```python
from build123d import *

# Parameters (mm, degrees)
F0_R     = 14.2875
F1_DEPTH = 14.2875
F2_R     = 6.35
F3_DEPTH = 44.45
F4_R     = 4.445
F5_DEPTH = 76.2


with BuildPart() as f1:
    # F0 (on Top) → F1 (new body, symmetric)
    with BuildSketch(Plane.XY):
        Circle(F0_R)
    extrude(amount=F1_DEPTH, both=True)

    # F2 (on face) → F3 (join)
    with BuildSketch(Plane(origin=(0, 0, -14.2875), x_dir=(1, 0, 0), z_dir=(0, 0, -1))):
        Circle(F2_R)
    extrude(amount=F3_DEPTH)

    # F4 (on Right) → F5 (join, symmetric)
    with BuildSketch(Plane.YZ):
        with Locations((0, -1.5875)):
            Circle(F4_R)
    extrude(amount=F5_DEPTH, both=True)

    # F6 (on Front) → F7 (revolve)
    with BuildSketch(Plane.XZ):
        with BuildLine():
            Line((-86.73837, -1.5875), (-66.41837, -1.5875))
            ThreePointArc((-66.41837, -1.5875), (-76.57837, 8.5725), (-86.73837, -1.5875))
        make_face()
        with BuildLine():
            ThreePointArc((86.73837, -1.5875), (76.57837, 8.5725), (66.41837, -1.5875))
            Line((66.41837, -1.5875), (86.73837, -1.5875))
        make_face()
    revolve(axis=Axis((-76.57837, 0, -1.5875), (-1, 0, 0)))


solid = f1.part
```
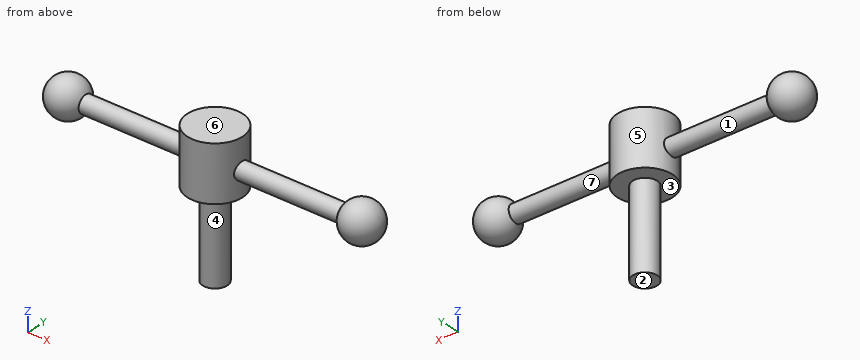
Here's how the part is built. I have some questions about the finished solid (model axes, mm). Face numbers are marked on the shaded views. A direction names the side the tool comes from. Coordinates: 2 decimals unless noted, no trailing zeros. Loops run counter-clockwise (first coordinate to the right, second up) from the corner with the lowest first, then second, coordinate; pieces in that order, holes last. Notation, with made-up numbers: M -24,-12 L 7,-12 A17 ccw 7,4 Z; hole C 59.25,-39 d4. An arc over 180 degrees is marked long. One line per item, written item: value.
1. On a 3-axis mill with a long thin cutter (end or side, diameter ignored), from which of +Z, -Z, +X, -X, +Y, -Y can I reach the whole of each face in a straight line? I mean the marked faces 1, 2 and 3. Say none if no direction works.
Geometry says:
face 1: none
face 2: -Z, +X, -X, +Y, -Y
face 3: -Z
2. Imagine slicing it at B-B (y = 0). List the corners of the cut face in (x, z) for me.
Geometry says:
outline: M -67.44,-6.03 L -14.29,-6.03 L -14.29,-14.29 L -6.35,-14.29 L -6.35,-58.74 L 6.35,-58.74 L 6.35,-14.29 L 14.29,-14.29 L 14.29,-6.03 L 67.44,-6.03 A10.16 ccw long 67.44,2.86 L 14.29,2.86 L 14.29,14.29 L -14.29,14.29 L -14.29,2.86 L -67.44,2.86 A10.16 ccw long Z
3. Imagine slicing it at A-A (x = 0). List the corners of the cut face in (y, z) for me.
Geometry says:
outline: M -14.29,-14.29 L -6.35,-14.29 L -6.35,-58.74 L 6.35,-58.74 L 6.35,-14.29 L 14.29,-14.29 L 14.29,14.29 L -14.29,14.29 Z
4. Imagine slicing it at C-C (z = -41). List the corners of the cut face in (x, y) for me.
Geometry says:
outline: C 0,0 d12.7
5. Thinking about a two-plate mould opening in X: for the marked faces 4, 5, 6 and 7, which applies, +X half, -X half, draft (parallel to the pull), parting line (faces both ways), or undercut?
Geometry says:
face 4: parting line
face 5: undercut
face 6: draft
face 7: undercut
6. Imagine slicing it at D-D (y = -8.25). List the corners of the cut face in (x, z) for me, and give its area (3 significant figures).
Geometry says:
outline: C -76.58,-1.59 d11.86; M -11.66,-14.29 L 11.66,-14.29 L 11.66,14.29 L -11.66,14.29 Z; C 76.58,-1.59 d11.86
area: 888 mm2
7. Will these pins go through, and if not, where does the flat tip stop? pin 1 Ø4 at (y, z) = (1, -1) entering from +X; pin 2 Ø4 at (y, z) = (-6.5, -18) entering from +X; pin 3 Ø1 at (y, z) = (-7, -2) entering from +X; pin 4 Ø1.5 at (x, z) = (-4, -45) entering from -Y.
Geometry says:
pin 1: stops at x = 86.74
pin 2: stops at x = 4.48
pin 3: stops at x = 84.38
pin 4: stops at y = -5.46
8. Please list where these lines run through material, in increasing order: probe 1 along Y at (x, z) = (0, -7.5); probe 2 along Y at (x, z) = (-1, -35).
Geometry says:
probe 1: y = -14.29 to 14.29
probe 2: y = -6.27 to 6.27
